from build123d import *

# Parameters (mm, degrees)
SKETCH1_W                 = 54.5
SKETCH1_H                 = 39
BOSS_EXTRUDE1_DEPTH       = 3
SKETCH10_R                = 7
CUT_EXTRUDE1_DEPTH        = 5
M2_CLEARANCE_HOLE1_D      = 2.4
M2_CLEARANCE_HOLE1_DEPTH  = 17
M2_CLEARANCE_HOLE1_TIP    = 0.721032743
SKETCH12_W                = 20
SKETCH12_H                = 5
BOSS_EXTRUDE2_DEPTH       = 28
SKETCH13_R                = 4.25
CUT_EXTRUDE2_DEPTH        = 5
SKETCH16_W                = 54.5
SKETCH16_H                = 5
BOSS_EXTRUDE4_DEPTH       = 12
F_8_CLEARANCE_HOLE1_D     = 4.4958
F_8_CLEARANCE_HOLE1_DEPTH = 17
F_8_CLEARANCE_HOLE1_TIP   = 1.350674586
RIB2_REACH                = 70.517
SKETCH20_WALL_W           = 166.493784704
SKETCH20_WALL_H           = 5
RIB4_REACH                = 70.517
SKETCH21_WALL_W           = 166.493784704
SKETCH21_WALL_H           = 5


with BuildPart() as part:
    # Sketch1 → Boss-Extrude1 (new body)
    with BuildSketch(Plane(origin=(0, 0, 0), x_dir=(1, 0, 0), z_dir=(0, 1, 0))):
        with Locations((-13.399543841, 8.129312584)):
            Rectangle(SKETCH1_W, SKETCH1_H)
    extrude(amount=BOSS_EXTRUDE1_DEPTH)

    # Sketch10 → Cut-Extrude1 (cut)
    with BuildSketch(Plane(origin=(0, 3, 0), x_dir=(1, 0, 0), z_dir=(0, 1, 0))):
        with Locations(Location((-10.149543841, 8.129312584, 0), (0, 0, 270))):
            Circle(SKETCH10_R)
    extrude(amount=-CUT_EXTRUDE1_DEPTH, mode=Mode.SUBTRACT)

    # M2 Clearance Hole1
    with Locations(Plane(origin=(-10.149543841, 3, -0.129312584), x_dir=(0, 0, 1), z_dir=(0, 1, 0))):
        with Locations((0, 0), (-8, 7.99475453), (-8, -7.99475453), (-16, 0)):
            Hole(M2_CLEARANCE_HOLE1_D / 2, depth=M2_CLEARANCE_HOLE1_DEPTH)
            with Locations((0, 0, -(M2_CLEARANCE_HOLE1_DEPTH + M2_CLEARANCE_HOLE1_TIP / 2))):  # 118° drill point
                Cone(0, M2_CLEARANCE_HOLE1_D / 2, M2_CLEARANCE_HOLE1_TIP, mode=Mode.SUBTRACT)

    # Sketch12 → Boss-Extrude2 (add)
    with BuildSketch(Plane(origin=(0, 3, 0), x_dir=(1, 0, 0), z_dir=(0, 1, 0))):
        with Locations((3.850456159, -8.870687416)):
            Rectangle(SKETCH12_W, SKETCH12_H)
        with Locations((-30.649543841, -8.870687416)):
            Rectangle(SKETCH12_W, SKETCH12_H)
    extrude(amount=BOSS_EXTRUDE2_DEPTH)

    # Sketch13 → Cut-Extrude2 (cut)
    with BuildSketch(Plane(origin=(0, 0, 6.370687416), x_dir=(-1, 0, 0), z_dir=(0, 0, -1))):
        with Locations((-3.850456159, 26)):
            Circle(SKETCH13_R)
        with Locations((30.649543841, 26)):
            Circle(SKETCH13_R)
    extrude(amount=-CUT_EXTRUDE2_DEPTH, mode=Mode.SUBTRACT)

    # Sketch16 → Boss-Extrude4 (add)
    with BuildSketch(Plane.XZ):
        with Locations((-13.399543841, 8.870687416)):
            Rectangle(SKETCH16_W, SKETCH16_H)
    extrude(amount=BOSS_EXTRUDE4_DEPTH)

    # #8 Clearance Hole1
    with Locations(Plane(origin=(-30.649543841, -8.2, 11.370687416), x_dir=(1, 0, 0), z_dir=(0, 0, 1))):
        with Locations((0, 0), (17.25, 0), (34.5, 0)):
            Hole(F_8_CLEARANCE_HOLE1_D / 2, depth=F_8_CLEARANCE_HOLE1_DEPTH)
            with Locations((0, 0, -(F_8_CLEARANCE_HOLE1_DEPTH + F_8_CLEARANCE_HOLE1_TIP / 2))):  # 118° drill point
                Cone(0, F_8_CLEARANCE_HOLE1_D / 2, F_8_CLEARANCE_HOLE1_TIP, mode=Mode.SUBTRACT)

    # Sketch20 wall → Rib2 (add, up to next)
    with BuildSketch(Plane(origin=(13.850456159, 14.5, -1.129312584), x_dir=(0, -0.837610596839, -0.546267780547), z_dir=(0, 0.546267780547, -0.837610596839)), mode=Mode.PRIVATE) as rib2_sk1:
        with Locations((0, 2.5)):
            Rectangle(SKETCH20_WALL_W, SKETCH20_WALL_H)
    rib2_tool1 = extrude(rib2_sk1.sketch, amount=-RIB2_REACH, mode=Mode.PRIVATE) - part.part
    add(rib2_tool1.solids().sort_by_distance((13.850456159, 14.5, -1.129312584))[0])

    # Sketch21 wall → Rib4 (add, up to next)
    with BuildSketch(Plane(origin=(-40.649543841, 14.5, -1.129312584), x_dir=(0, -0.837610596839, -0.546267780547), z_dir=(0, -0.546267780547, 0.837610596839)), mode=Mode.PRIVATE) as rib4_sk1:
        with Locations((0, 2.5)):
            Rectangle(SKETCH21_WALL_W, SKETCH21_WALL_H)
    rib4_tool1 = extrude(rib4_sk1.sketch, amount=RIB4_REACH, mode=Mode.PRIVATE) - part.part
    add(rib4_tool1.solids().sort_by_distance((-40.649543841, 14.5, -1.129312584))[0])


solid = part.part
Model file for the job. Use its own axes, mm. A direction names the side the tool comes from. Give positions to 0.01 mm unless a question says otherwise; leave off trailing zeros. Order: outer loops, then holes, each group sorted by start corner. A loop starts at its lowest first (then second) coordinate and runs counter-clockwise, first axis right, second up. Notation, with made-up numbers: M -9.5,-8 L 41.5,-8 A12 ccw 41.5,13 Z; hole C -29.75,-8.5 d11. An arc over 180 degrees is marked long. Put each result on its own line as item: value. Start each with the question number.
(1) Band-saw the part on C-C on y = 7.5. Give the cut face in (x, z), then the cut area to 3 significant figures.
(2) Pin check, flat tips, straight feed: pin 1 Ø5 at (x, y) = (3.85, -8.2) entering from -Z; pin 2 Ø8 at (x, z) = (-2.5, -10) entering from +Y; pin 3 Ø3 at (x, z) = (-10.15, -0.13) entering from -Y. Stop position of each tip, or through.
(3) Pull direction Z, two halves, no side cores. Call faces 1 (the face through (-10.19, 1.48, -17.33)), 2 (the face through (-40.65, 8, 4)), 3 (the face through (11.3, 14.7, -1)): released by +Z, released by -Z, zero draft, split by the parting line, or undercut.
(4) Tool access for faces 4 (the face through (-5.25, 1.52, -3.13)), 5 (the face through (8.85, 9, 1)), 6 (the face through (-31, 31, 9)), 7 (the face through (-27.517, 28.872, 8.836)), 8 (the face through (-20.65, 17, 9)): list every direction of +Z, -Z, +X, -X, +Y, -Y with a clear straight run to the whole face (end or side of a thin tool).
(5) Band-saw the part on A-A on y = -8.2. Give the cut face in (x, z), then the cut area to 3 significant figures.
(6) Band-saw the part on D-D on x = -24. Give the cut face in (y, z).
(7) Band-saw the part on B-B on x = -34. Give the cut face in (y, z).
(8) Drill centre lines: L1, parallel to X at y = 13, z = 4; L2, parallel to Y at x = -4, z = -21; L3, parallel to Z at x = -32.5, y = 20.5. Where is each one in solid material? Low to high. Write a range as [from, to].
Results below:
1. outline: M -40.65,-5.69 L -35.65,-5.69 L -35.65,6.37 L -20.65,6.37 L -20.65,11.37 L -40.65,11.37 Z; M -6.15,6.37 L 8.85,6.37 L 8.85,-5.69 L 13.85,-5.69 L 13.85,11.37 L -6.15,11.37 Z
1. area: 321 mm2
2. pin 1: stops at z = 6.37
2. pin 2: stops at y = 3
2. pin 3: stops at y = 0
3. face 1: undercut
3. face 2: zero draft
3. face 3: released by -Z
4. face 4: +Y, -Y
4. face 5: -Z, +Y
4. face 6: +Z, -Z, +X, -X, +Y
4. face 7: +Z, -Z
4. face 8: +Z, -Z, +Y
5. outline: M -40.65,6.37 L -32.9,6.37 L -32.9,11.37 L -40.65,11.37 Z; M -28.4,6.37 L -15.65,6.37 L -15.65,11.37 L -28.4,11.37 Z; M -11.15,6.37 L 1.6,6.37 L 1.6,11.37 L -11.15,11.37 Z; M 6.1,6.37 L 13.85,6.37 L 13.85,11.37 L 6.1,11.37 Z
5. area: 205 mm2
6. outline: M -12,6.37 L 0,6.37 L 0,-27.63 L 3,-27.63 L 3,6.37 L 31,6.37 L 31,11.37 L -12,11.37 Z
7. outline: M -12,6.37 L 0,6.37 L 0,-27.63 L 3,-27.63 L 3,6.37 L 23.39,6.37 L 23.39,11.37 L -12,11.37 Z; M 28.61,6.37 L 31,6.37 L 31,11.37 L 28.61,11.37 Z
8. L1: x = [-40.65, -35.65], [8.85, 13.85]
8. L2: y = [0, 3]
8. L3: z = [6.37, 11.37]
